Input: dimensioned drawing with shaded views. Units: mm. Origin: part minimum x, y, z. Coordinates: 2 decimals unless noted, no trailing zeros. Order: outer loops, then holes, each group sorted by start corner. A loop starts at its lowest first (then second) coordinate and runs counter-clockwise, first axis right, second up.
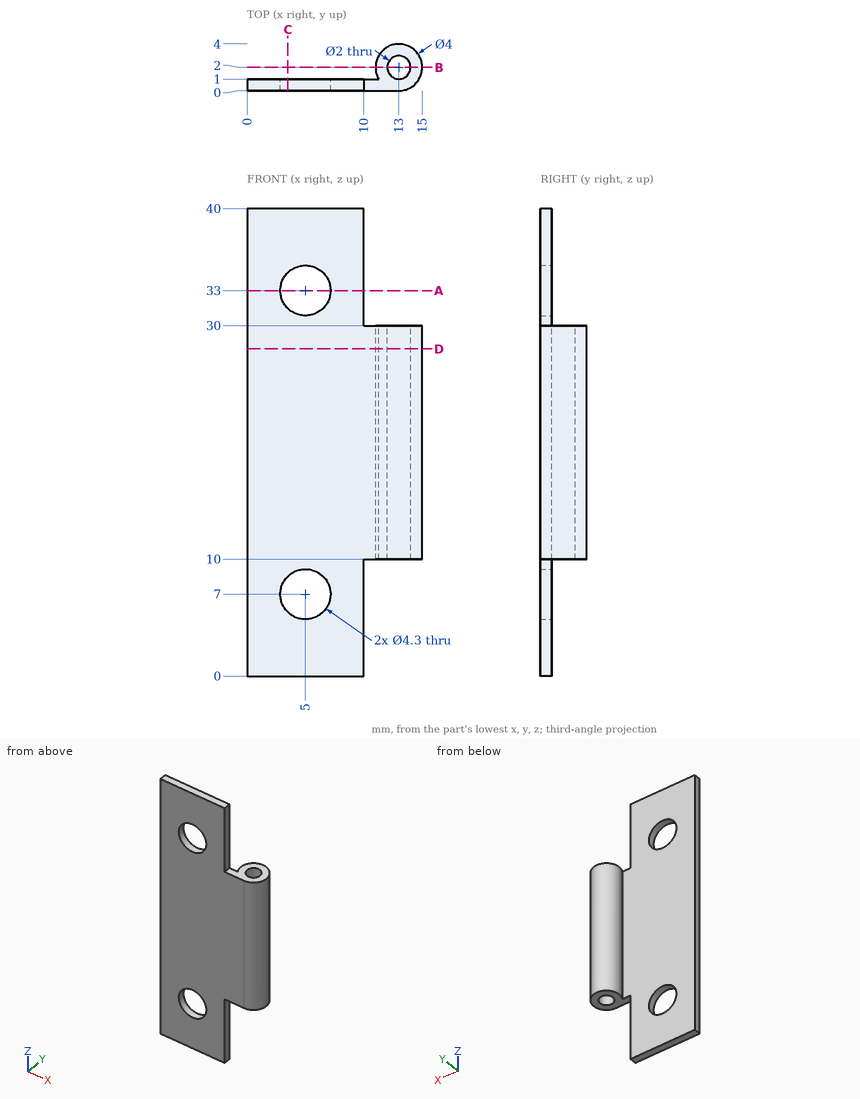
1. Section query C-C on x = 3.5. Return loops of the section in (y, z), plus the area to 3 significant figures.
Findings:
outline: (0, 0) - (1, 0) - (1, 5.46) - (0, 5.46) - close; (0, 8.54) - (1, 8.54) - (1, 31.46) - (0, 31.46) - close; (0, 34.54) - (1, 34.54) - (1, 40) - (0, 40) - close
area: 33.8 mm2
2. Ray query, line 1 (Z direction, x = 6, y = 0.4); line 2 (Y direction, x = 2, z = 30); line 3 (X direction, y = 1.7, z = 26.5). Return the intervals inside material, ascending.
Findings:
line 1: z = 0 to 5.1, 8.9 to 31.1, 34.9 to 40
line 2: y = 0 to 1
line 3: x = 11.02 to 12.05, 13.95 to 14.98
3. Pin query (flat end, axial travel): P1, Ø1.1, axis at y = 0.5, z = 37, coming from the +X side; P2, Ø5.5, axis at x = 8, z = 23, coming from the +Y side; P3, Ø1.2, axis at x = 12, y = 1.5, coming from the -Z side. Return the tip coordinate at first contact, or that it passes through.
Findings:
P1: stops at x = 10
P2: stops at y = 1
P3: stops at z = 10
4. Section query B-B on y = 2. Return loops of the section in (x, z).
Findings:
outline: (11, 10) - (12, 10) - (12, 30) - (11, 30) - close; (14, 10) - (15, 10) - (15, 30) - (14, 30) - close
5. Section query A-A on z = 33. Return loops of the section in (x, y).
Findings:
outline: (0, 0) - (2.85, 0) - (2.85, 1) - (0, 1) - close; (7.15, 0) - (10, 0) - (10, 1) - (7.15, 1) - close
6. Section query D-D on z = 28. Return loops of the section in (x, y), plus the area to 3 significant figures.
Findings:
outline: (0, 0) - (13, 0) arc R2 ccw (long way) to (11.27, 1) - (0, 1) - close; hole circle Ø2 at (13, 2)
area: 21.2 mm2
